The listing builds one solid part. Answer for the finished solid, in the listing's coordinates (mm). Round coordinates to 2 decimals unless told otherwise and drop trailing zeros. Write each loop counter-clockwise with the first axis right and the second up, starting at its lowest first coordinate (ties: lowest second). Pieces come first, ordered by that corner, then holes. Notation, with made-up numbers: (8.25, -24) -> (52.25, -24) arc R14 cw to (52.25, -9) -> close; hole circle Ø11 at (50.5, -14). An arc over 180 degrees is marked (long way). Write each question's results on one line, items separated by ' | '. Start each with the question number.
```python
from build123d import *

# Parameters (mm, degrees)
F0_R     = 1.65
F1_DEPTH = 4


with BuildPart() as f1:
    # F0 (on Top) → F1 (new body)
    with BuildSketch(Plane.XY):
        with BuildLine():
            Line((-20, 34.1743044555), (-20, 20))
            Line((-20, 20), (-20, 9.0556954967))
            Line((-20, 9.0556954967), (-20, -7.4999716698))
            Line((-20, -7.4999716698), (-20, -20))
            Line((-20, -20), (-20, -31))
            Line((-20, -31), (-14.9161266072, -31))
            Line((-14.9161266072, -31), (-8.6228793733, -23.5))
            Line((-8.6228793733, -23.5), (-10, -23.5))
            ThreePointArc((-10, -23.5), (-11.75, -21.75), (-10, -20))
            Line((-10, -20), (-5.6860306642, -20))
            Line((-5.6860306642, -20), (4.3806233749, -20))
            Line((4.3806233749, -20), (10, -20))
            ThreePointArc((10, -20), (11.2374368671, -20.5125631329), (11.75, -21.75))
            ThreePointArc((11.75, -21.75), (11.2374368671, -22.9874368671), (10, -23.5))
            Line((10, -23.5), (7.317472084, -23.5))
            Line((7.317472084, -23.5), (13.6107193178, -31))
            Line((13.6107193178, -31), (20, -31))
            Line((20, -31), (20, -20))
            Line((20, -20), (20, -9.0556954967))
            Line((20, -9.0556954967), (20, 9.0556954967))
            Line((20, 9.0556954967), (20, 20))
            Line((20, 20), (20, 34.1743044555))
            Line((20, 34.1743044555), (16.2742770157, 34.1743044555))
            Line((16.2742770157, 34.1743044555), (14.5960777534, 32.1743044555))
            Line((14.5960777534, 32.1743044555), (16, 32.1743044555))
            Line((16, 32.1743044555), (16, 28.6743044555))
            Line((16, 28.6743044555), (14, 28.6743044555))
            Line((14, 28.6743044555), (14, 31.4639266515))
            Line((14, 31.4639266515), (7.317472084, 23.5))
            Line((7.317472084, 23.5), (10, 23.5))
            ThreePointArc((10, 23.5), (11.2374368671, 22.9874368671), (11.75, 21.75))
            ThreePointArc((11.75, 21.75), (11.2374368671, 20.5125631329), (10, 20))
            Line((10, 20), (0, 20))
            Line((0, 20), (-4.3806233749, 20))
            Line((-4.3806233749, 20), (-10, 20))
            ThreePointArc((-10, 20), (-11.75, 21.75), (-10, 23.5))
            Line((-10, 23.5), (-7.317472084, 23.5))
            Line((-7.317472084, 23.5), (-14, 31.4639266515))
            Line((-14, 31.4639266515), (-14, 28.6743044555))
            Line((-14, 28.6743044555), (-16, 28.6743044555))
            Line((-16, 28.6743044555), (-16, 32.1743044555))
            Line((-16, 32.1743044555), (-14.5960777534, 32.1743044555))
            Line((-14.5960777534, 32.1743044555), (-16.2742770157, 34.1743044555))
            Line((-16.2742770157, 34.1743044555), (-20, 34.1743044555))
        make_face()
        with Locations((-15.25, -15.25)):
            Circle(F0_R, mode=Mode.SUBTRACT)
        with Locations((15.25, -15.25)):
            Circle(F0_R, mode=Mode.SUBTRACT)
        with Locations((-15.25, 15.25)):
            Circle(F0_R, mode=Mode.SUBTRACT)
        with Locations((15.25, 15.25)):
            Circle(F0_R, mode=Mode.SUBTRACT)
        with BuildLine():
            Line((-20, 9.0556954967), (-20, 20))
            Line((-20, 20), (-20, 34.1743044555))
            Line((-20, 34.1743044555), (-16.2742770157, 34.1743044555))
            Line((-16.2742770157, 34.1743044555), (-65.6094303769, 92.9696507149))
            ThreePointArc((-65.6094303769, 92.9696507149), (-70.7066370655, 84.2648887431), (-80.1642747962, 80.7566861309))
            Line((-80.1642747962, 80.7566861309), (-20, 9.0556954967))
        make_face()
        with BuildLine():
            Line((-20, -20), (-20, -7.4999716698))
            Line((-20, -7.4999716698), (-81.5062852996, -80.8003081427))
            ThreePointArc((-81.5062852996, -80.8003081427), (-71.7350386168, -83.4751187737), (-65.8927282585, -91.7515481563))
            Line((-65.8927282585, -91.7515481563), (-14.9161266072, -31))
            Line((-14.9161266072, -31), (-20, -31))
            Line((-20, -31), (-20, -20))
        make_face()
        with BuildLine():
            ThreePointArc((-65.3484512108, 95.7555553899), (-91.0199704611, 106.2968397941), (-80.1642747962, 80.7566861309))
            Line((-80.1642747962, 80.7566861309), (-87.6258734204, 89.6490730979))
            Line((-87.6258734204, 89.6490730979), (-80.3484512108, 95.7555553899))
            Line((-80.3484512108, 95.7555553899), (-73.0710290012, 101.8620376819))
            Line((-73.0710290012, 101.8620376819), (-65.6094303769, 92.9696507149))
            ThreePointArc((-65.6094303769, 92.9696507149), (-65.413838519, 94.3565043737), (-65.3484512108, 95.7555553899))
        make_face()
        with BuildLine():
            Line((-87.6258734204, 89.6490730979), (-80.1642747962, 80.7566861309))
            ThreePointArc((-80.1642747962, 80.7566861309), (-70.7066370655, 84.2648887431), (-65.6094303769, 92.9696507149))
            Line((-65.6094303769, 92.9696507149), (-73.0710290012, 101.8620376819))
            Line((-73.0710290012, 101.8620376819), (-80.3484512108, 95.7555553899))
            Line((-80.3484512108, 95.7555553899), (-87.6258734204, 89.6490730979))
        make_face()
        Polygon((16.2742770157, 34.1743044555), (-16.2742770157, 34.1743044555), (-14.5960777534, 32.1743044555), (-14, 32.1743044555), (-14, 31.4639266515), (-7.317472084, 23.5), (7.317472084, 23.5), (14, 31.4639266515), (14, 32.1743044555), (14.5960777534, 32.1743044555), align=None)
        with BuildLine():
            ThreePointArc((-65.8927282585, -91.7515481563), (-71.7350386168, -83.4751187737), (-81.5062852996, -80.8003081427))
            Line((-81.5062852996, -80.8003081427), (-88.3919178636, -89.0062854882))
            Line((-88.3919178636, -89.0062854882), (-80.3484512108, -95.7555553899))
            Line((-80.3484512108, -95.7555553899), (-73.8370734443, -101.2192500722))
            Line((-73.8370734443, -101.2192500722), (-65.8927282585, -91.7515481563))
        make_face()
        with BuildLine():
            Line((-88.3919178636, -89.0062854882), (-81.5062852996, -80.8003081427))
            ThreePointArc((-81.5062852996, -80.8003081427), (-90.5374768921, -106.7639047514), (-65.3484512108, -95.7555553899))
            ThreePointArc((-65.3484512108, -95.7555553899), (-65.485143297, -93.7351401212), (-65.8927282585, -91.7515481563))
            Line((-65.8927282585, -91.7515481563), (-73.8370734443, -101.2192500722))
            Line((-73.8370734443, -101.2192500722), (-80.3484512108, -95.7555553899))
            Line((-80.3484512108, -95.7555553899), (-88.3919178636, -89.0062854882))
        make_face()
        with BuildLine():
            Line((65.6094303769, 92.9696507149), (16.2742770157, 34.1743044555))
            Line((16.2742770157, 34.1743044555), (20, 34.1743044555))
            Line((20, 34.1743044555), (20, 20))
            Line((20, 20), (20, 9.0556954967))
            Line((20, 9.0556954967), (80.1642747962, 80.7566861309))
            ThreePointArc((80.1642747962, 80.7566861309), (70.7066370655, 84.2648887431), (65.6094303769, 92.9696507149))
        make_face()
        with BuildLine():
            ThreePointArc((95.3484512108, 95.7555553899), (78.9494001947, 110.6901680817), (65.6094303769, 92.9696507149))
            Line((65.6094303769, 92.9696507149), (73.0710290012, 101.8620376819))
            Line((73.0710290012, 101.8620376819), (80.3484512108, 95.7555553899))
            Line((80.3484512108, 95.7555553899), (87.6258734204, 89.6490730979))
            Line((87.6258734204, 89.6490730979), (80.1642747962, 80.7566861309))
            ThreePointArc((80.1642747962, 80.7566861309), (90.889735615, 85.0840361396), (95.3484512108, 95.7555553899))
        make_face()
        with BuildLine():
            Line((73.0710290012, 101.8620376819), (65.6094303769, 92.9696507149))
            ThreePointArc((65.6094303769, 92.9696507149), (70.7066370655, 84.2648887431), (80.1642747962, 80.7566861309))
            Line((80.1642747962, 80.7566861309), (87.6258734204, 89.6490730979))
            Line((87.6258734204, 89.6490730979), (80.3484512108, 95.7555553899))
            Line((80.3484512108, 95.7555553899), (73.0710290012, 101.8620376819))
        make_face()
        Polygon((-8.6228793733, -23.5), (-14.9161266072, -31), (13.6107193178, -31), (7.317472084, -23.5), align=None)
        with BuildLine():
            Line((20, -31), (13.6107193178, -31))
            Line((13.6107193178, -31), (65.6094303769, -92.9696507149))
            ThreePointArc((65.6094303769, -92.9696507149), (70.7066370655, -84.2648887431), (80.1642747962, -80.7566861309))
            Line((80.1642747962, -80.7566861309), (20, -9.0556954967))
            Line((20, -9.0556954967), (20, -20))
            Line((20, -20), (20, -31))
        make_face()
        with BuildLine():
            ThreePointArc((80.1642747962, -80.7566861309), (70.7066370655, -84.2648887431), (65.6094303769, -92.9696507149))
            Line((65.6094303769, -92.9696507149), (73.0710290012, -101.8620376819))
            Line((73.0710290012, -101.8620376819), (80.3484512108, -95.7555553899))
            Line((80.3484512108, -95.7555553899), (87.6258734204, -89.6490730979))
            Line((87.6258734204, -89.6490730979), (80.1642747962, -80.7566861309))
        make_face()
        with BuildLine():
            Line((73.0710290012, -101.8620376819), (65.6094303769, -92.9696507149))
            ThreePointArc((65.6094303769, -92.9696507149), (78.9494001947, -110.6901680817), (95.3484512108, -95.7555553899))
            ThreePointArc((95.3484512108, -95.7555553899), (90.889735615, -85.0840361396), (80.1642747962, -80.7566861309))
            Line((80.1642747962, -80.7566861309), (87.6258734204, -89.6490730979))
            Line((87.6258734204, -89.6490730979), (80.3484512108, -95.7555553899))
            Line((80.3484512108, -95.7555553899), (73.0710290012, -101.8620376819))
        make_face()
    extrude(amount=F1_DEPTH)


solid = f1.part
```
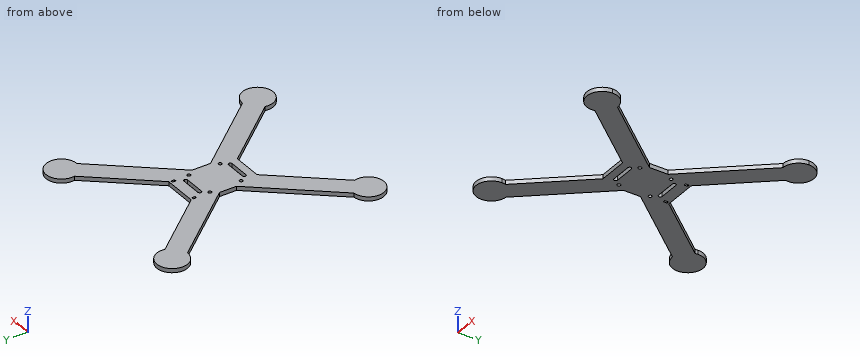
Q1. Each of these flat-tipped pins is pushed along its axis until it touches: pin 1 (1.5 mm diameter, centred on x = 31.5, z = 2, fed in from +Y); pin 2 (1 mm diameter, centred on y = 30.5, z = 2.5, fed in from -X); pin 3 (1 mm diameter, centred on x = 61.5, z = 3, fed in from +Y); pin 4 (4 mm diameter, centred on x = -15.25, y = -15.25, fed in from +Z). Where does it stop, or does it pass through?
Q2. The part is cut by section A-A, the plane y = -52. Write down the section's boundary in (x, z), then the cut area to 3 significant figures.
Q3. The part is cut by section C-C, the plane z = 0.6. State how many separate pieces and enclosed holes the cut face has, then the cut area to 3 significant figures.
Q4. The part is cut by section D-D, the plane y = 4. Write down the section's boundary in (x, z).
Q5. The part is cut by section B-B, the plane x = 24.5. Write down the section's boundary in (y, z).
Q6. Find the intervals of material crossed by line 1 (Y direction, x = -15.25, z = 1.6); line 2 (Y direction, x = 15.25, z = 0.95); line 3 (X direction, y = 89.5, z = 2.8), in increasing order.
Answers follow:
1) pin 1: y = 53.21 | pin 2: x = -38.41 | pin 3: y = 88.67 | pin 4: z = 4
2) outline: (-57.34, 0) -> (-32.54, 0) -> (-32.54, 4) -> (-57.34, 4) -> close; (31.23, 0) -> (56.03, 0) -> (56.03, 4) -> (31.23, 4) -> close | area: 198 mm^2
3) separate pieces: 1 | enclosed holes: 8 | area: 11,400 mm^2
4) outline: (-20, 0) -> (20, 0) -> (20, 4) -> (-20, 4) -> close
5) outline: (-43.98, 0) -> (-14.42, 0) -> (-14.42, 4) -> (-43.98, 4) -> close; (14.42, 0) -> (43.98, 0) -> (43.98, 4) -> (14.42, 4) -> close
6) line 1: -31.4 to -16.9, -13.6 to 13.6, 16.9 to 28.67, 32.17 to 34.17 | line 2: -32.95 to -16.9, -13.6 to 13.6, 16.9 to 28.67, 32.17 to 34.17 | line 3: -93.98 to -62.7, 62.7 to 93.98
